Source: CAD feature listing. Evaluate the final solid. Frame: model axes, mm. Face numbers are marked on the shaded views. A direction names the side the tool comes from. Coordinates: 2 decimals unless noted, no trailing zeros. Order: outer loops, then holes, each group sorted by start corner. A loop starts at its lowest first (then second) coordinate and runs counter-clockwise, first axis right, second up. Notation, with made-up numbers: (28.5, 11) -> (81.5, 11) arc R38 cw to (81.5, 49) -> close; hole circle Ø9 at (82.25, -31.5). An arc over 180 degrees is marked (long way). Put each result on its own line as item: value.
Autodesk Inventor part; units mm, degrees
ref_plane "YZ Plane" through (0, 0, 0) normal (1, 0, 0) x (0, 1, 0)
ref_plane "XZ Plane" through (0, 0, 0) normal (0, 1, 0) x (-1, 0, 0)
ref_plane "XY Plane" through (0, 0, 0) normal (0, 0, 1) x (1, 0, 0)
sketch "Boceto1" plane through (0, 0, 0) normal (0, 1, 0) x (-1, 0, 0)
  circle A0 centre (0, 0) radius 14
  dimension "d0" = 28
extrude "Extrusión1" add sketch "Boceto1" along normal blind 60
shell "Vaciado1" thickness 2 removed faces 1 at (-2.651, 60, 3.8406)
sketch "Boceto2" plane through (0, 0, 0) normal (1, 0, 0) x (0, 1, 0)
  line L0 (0, -14) -> (60, -14)
  line L1 (0, 14) -> (60, 14)
  line L2 (46, -14) -> (48, -14)
  line L3 (48, -14) -> (48, -19)
  line L4 (48, -19) -> (46, -19)
  line L5 (46, -19) -> (46, -14)
  point P0 (0, 0)
  dimension "d4" = 14
  dimension "d5" = 2
  dimension "d6" = 5
sketch "Boceto3" plane through (0, 0, 0) normal (1, 0, 0) x (0, 1, 0)
  line L0 (84.0119, 0) -> (36.1853, 0)
  point P0 (0, 0)
sketch "Boceto4" plane through (0, 0, 0) normal (0, -1, 0) x (1, 0, 0)
  circle A0 centre (0, 0) radius 3
  circle A1 centre (0, 0) radius 6
  dimension "d7" = 6
  dimension "d8" = 12
extrude "Extrusión2" cut sketch "Boceto4" against normal through all contours A0
sketch "Boceto5" plane through (0, 0, 0) normal (0, -1, 0) x (1, 0, 0)
  circle A0 centre (0, 0) radius 3
sketch "Boceto6" plane through (0, 0, 0) normal (0, 0, 1) x (1, 0, 0)
  line L0 (-14, 0) -> (-14, 60)
  line L1 (-14, 42) -> (-18, 42)
  line L2 (-18, 42) -> (-18, 40)
  line L3 (-18, 40) -> (-14, 40)
  line L4 (14, 60) -> (-14, 60)
  line L5 (0, -14.2107) -> (0, 116.483)
  point P0 (0, 0)
  dimension "d11" = 18
  dimension "d12" = 2
  dimension "d13" = 4
sketch "Boceto7" plane through (0, 0, 0) normal (0, -1, 0) x (1, 0, 0)
  circle A0 centre (0, 0) radius 3
  circle A1 centre (0, 0) radius 8
  dimension "d14" = 16
extrude "Extrusión3" add sketch "Boceto7" along normal blind 6
sketch "Boceto8" plane through (0, -6, 0) normal (0, -1, 0) x (1, 0, 0)
  circle A0 centre (0, 0) radius 8
  circle A1 centre (0, 0) radius 6
  circle A2 centre (0, 0) radius 3
  dimension "d17" = 2
extrude "Extrusión4" cut sketch "Boceto8" against normal blind 4 contours A1
chamfer "Chaflán1" distance 1.5 angle 45 1 edges at (-6, -6, 0)
revolve "Revolución1" add sketch "Boceto6" angle 360 about axis through (0, -14.2107, 0) along (0, 1, 0)
chamfer "Chaflán2" distance 0.5 angle 45 2 edges at (18, 40, 0) (18, 42, 0)
properties part number "shocks_spring" material "Plata"
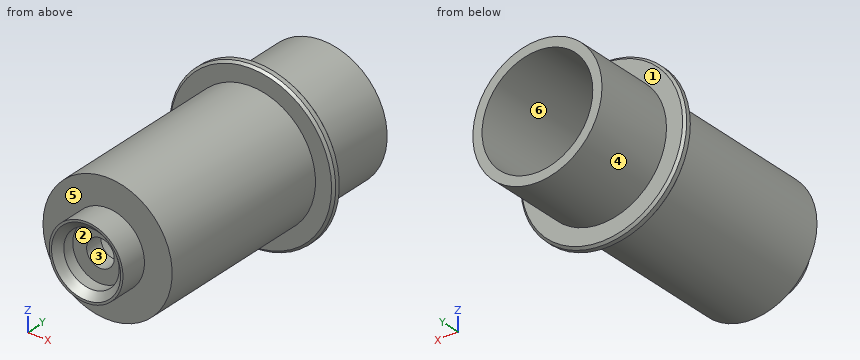
1. First-contact query: pin 1 (5 mm diameter, centred on y = 20, z = 10.5, fed in from -X); pin 2 (1.5 mm diameter, centred on y = 29.5, z = -5, fed in from -X); pin 3 (5 mm diameter, centred on y = 34, z = -14, fed in from -X); pin 4 (5 mm diameter, centred on x = 0, z = 0, fed in from -Y). Flat tips, straight axial feed; report the tip coordinate or a pass-through.
Numbers:
pin 1: stops at x = -11.49
pin 2: stops at x = -13.34
pin 3: stops at x = -7.98
pin 4: passes through
2. Pull-direction query (Z, two-part tool) for the marked faces 4, 5 and 6; classes: pulls with the +Z half, pulls with the -Z half, needs draft (parallel to the pull), parting line crosses it, or undercut.
Numbers:
face 4: parting line crosses it
face 5: needs draft
face 6: undercut
3. Cut plane C-C on y = 28.5. Output: boundary loops of the cut face in (x, z).
Numbers:
outline: circle Ø28 at (0, 0); hole circle Ø24 at (0, 0)
4. Set-up query: the marked faces 1, 2 and 3. Return all of +Z, -Z, +X, -X, +Y, -Y with unobstructed straight access to the full face (end or side cutting, diameter ignored); none if empty.
Numbers:
face 1: +Y
face 2: -Y
face 3: +Y, -Y
5. Ray query, line 1 along Z through (x, y) = (0, -2.45); line 2 along Z through (x, y) = (0, 34); line 3 along X through (y, z) = (13, -0.5). Return the intervals inside material, ascending.
Numbers:
line 1: z = -8 to -6, 6 to 8
line 2: z = -14 to -12, 12 to 14
line 3: x = -13.99 to -11.99, 11.99 to 13.99
